For this review, take the finished solid that the model builds, in its own axes (mm). A direction names the side the tool comes from. Coordinates: 2 decimals unless noted, no trailing zeros. Write each loop counter-clockwise with the first axis right and the second up, starting at its lowest first coordinate (ties: lowest second). Pieces come first, ordered by that corner, then holes.
```python
from build123d import *

# Parameters (mm, degrees)
SKETCH2_W             = 3.175
SKETCH2_H             = 4.572
BOSS_EXTRUDE1_DEPTH   = 0.762
SKETCH2_W_2           = 3.302
BOSS_EXTRUDE1_2_DEPTH = 0.762
BOSS_EXTRUDE2_DEPTH   = 0.7366
FILLET1_R             = 0.254
SKETCH4_W             = 3.429
SKETCH4_H             = 4.826
BOSS_EXTRUDE3_DEPTH   = 0.381


with BuildPart() as part:
    # Sketch2 → Boss-Extrude1 (new body)
    with BuildSketch(Plane.XY):
        Rectangle(SKETCH2_W, SKETCH2_H)
    extrude(amount=BOSS_EXTRUDE1_DEPTH)



with BuildPart() as body_2:
    # Sketch2 → Boss-Extrude1 2 (new body)
    with BuildSketch(Plane.XY):
        with Locations((3.937, 0)):
            Rectangle(SKETCH2_W_2, SKETCH2_H)
    extrude(amount=BOSS_EXTRUDE1_2_DEPTH)


with BuildPart() as part_1:
    add(part.part)

    add(body_2.part)  # Boss-Extrude2 merges body 2
    # Sketch3 → Boss-Extrude2 (add)
    with BuildSketch(Plane.XY):
        Polygon((-1.5875, -2.286), (1.5875, -2.286), (2.286, -2.286), (5.588, -2.286), (5.588, 2.286), (2.286, 2.286), (1.5875, 2.286), (-1.5875, 2.286), align=None)
    extrude(amount=-BOSS_EXTRUDE2_DEPTH)

    # Fillet1
    fillet1_edges = [part_1.edges().sort_by_distance(p)[0] for p in [
        (2.00025, 2.286, -0.7366),
        (5.588, 0, -0.7366),
        (2.00025, -2.286, -0.7366),
        (-1.5875, 0, -0.7366),
    ]]
    fillet(fillet1_edges, radius=FILLET1_R)

    # Sketch4 → Boss-Extrude3 (add)
    with BuildSketch(Plane.XY.offset(0.762)):
        Rectangle(SKETCH4_W, SKETCH4_H)
        with Locations((3.937, 0)):
            Rectangle(SKETCH4_W, SKETCH4_H)
    extrude(amount=-BOSS_EXTRUDE3_DEPTH)


solid = part_1.part
```
Q1. Add section A-A (z = 0.15). State the section outline as (x, y) points.
Ans:
outline: (-1.59, -2.29) - (1.59, -2.29) - (1.59, 2.29) - (-1.59, 2.29) - close; (2.29, -2.29) - (5.59, -2.29) - (5.59, 2.29) - (2.29, 2.29) - close
Q2. Draft analysis for pull direction X (two halves, no side actions). For faces 4 (the flat face through (-1.588, 0, 0)), 5 (the flat face through (5.588, 0, 0)), 6 (the flat face through (2, 0, -0.737)), state which applies: +X half, -X half, draft (parallel to the pull), parting line (faces both ways), or undercut.
Ans:
face 4: -X half
face 5: +X half
face 6: draft
Q3. Add section D-D (z = 0.55). State the section outline as (x, y) points, then the cut area to 3 significant figures.
Ans:
outline: (-1.71, -2.41) - (1.71, -2.41) - (1.71, 2.41) - (-1.71, 2.41) - close; (2.22, -2.41) - (5.65, -2.41) - (5.65, 2.41) - (2.22, 2.41) - close
area: 33.1 mm2
Q4. For probe 1 along X at (y, z) = (-2, 0.05); probe 2 along X at (y, z) = (1.1, 0.65); probe 3 along Y at (x, z) = (2.25, -0.3), list the stretches that pass through material, from the lowest coordinate up.
Ans:
probe 1: x = -1.59 to 1.59, 2.29 to 5.59
probe 2: x = -1.71 to 1.71, 2.22 to 5.65
probe 3: y = -2.29 to 2.29
Q5. Tool access review of faces 1 (the flat face through (4, 0, 0.762)), 2 (the flat face through (2.1, 2.286, -0.2)), 3 (the flat face through (2, -2.286, -0.2)): name each direction out of +Z, -Z, +X, -X, +Y, -Y from which nothing blocks a thin tool from reaching the whole face with its end or side.
Ans:
face 1: +Z, +X, -X, +Y, -Y
face 2: -Z, +X, -X, +Y
face 3: -Z, +X, -X, -Y
Q6. Add section B-B (x = 3.25). State the section outline as (y, z) points, then the cut area to 3 significant figures.
Ans:
outline: (-2.41, 0.38) - (-2.29, 0.38) - (-2.29, -0.48) arc R0.25 ccw to (-2.03, -0.74) - (2.03, -0.74) arc R0.25 ccw to (2.29, -0.48) - (2.29, 0.38) - (2.41, 0.38) - (2.41, 0.76) - (-2.41, 0.76) - close
area: 6.92 mm2
Q7. Add section C-C (y = 1.65). State the section outline as (x, z) points, then the cut area to 3 significant figures.
Ans:
outline: (-1.71, 0.38) - (-1.59, 0.38) - (-1.59, -0.48) arc R0.25 ccw to (-1.33, -0.74) - (5.33, -0.74) arc R0.25 ccw to (5.59, -0.48) - (5.59, 0.38) - (5.65, 0.38) - (5.65, 0.76) - (2.22, 0.76) - (2.22, 0.38) - (2.29, 0.38) - (2.29, 0) - (1.59, 0) - (1.59, 0.38) - (1.71, 0.38) - (1.71, 0.76) - (-1.71, 0.76) - close
area: 10.3 mm2
